Build history of the part. All positions in model axes, mm. Face numbers are marked on the shaded views. A direction names the side the tool comes from. Round coordinates to 2 decimals unless told otherwise and drop trailing zeros. Write each loop counter-clockwise with the first axis right and the second up, starting at its lowest first coordinate (ties: lowest second). Pieces come first, ordered by that corner, then holes. Notation, with made-up numbers: (83.5, 0) - (136.5, 0) arc R15 cw to (136.5, 24) - close; hole circle Ø3 at (53.25, -12.75). An arc over 180 degrees is marked (long way). Answer as a JSON object with one key per item and string values. Group by question number.
Item 1: Flat gauge pins, fed straight in: pin 1 (0.5 mm diameter, centred on y = 5.5, z = 0, fed in from +X); pin 2 (1.2 mm diameter, centred on x = -4, z = 1, fed in from -Y); pin 3 (1.5 mm diameter, centred on x = -3.5, y = 3.5, fed in from -Z). Where does each tip first touch, or does it go through?
Item 2: Which spindle directions (+Z, -Z, +X, -X, +Y, -Y) get a long thin tool onto all of the face, cutting with end or side? Do the marked faces 1, 2, 3 and 4. Say none if no direction does.
Item 3: Slice it at A-A, the plane x = -4.6. List the corners of the cut face in (y, z).
Item 4: Slice it at B-B, the plane y = -3.75. List the corners of the cut face in (x, z).
Item 5: Slice it at C-C, the plane z = -1.65. List the corners of the cut face in (x, y), then the cut area to 3 significant figures.
Item 6: Two-plate mould, pull along Y, no slides. Class the marked faces 5, 6 and 7: +Y half, -Y half, draft (parallel to the pull), parting line (faces both ways), or undercut.
Item 7: Probe line 1 (X direction, y = -3.7, z = 0); line 2 (Y direction, x = 0, z = 1.25); line 3 (Y direction, x = -3.25, z = 0.8). List the from-to ranges inside material, lowest first. Write a range as from..to.
Item 8: Slice it at D-D, the plane x = 0. List the corners of the cut face in (y, z).
from build123d import *

# Parameters (mm, degrees)
EXTRUDE_1_DEPTH      = 4
EXTRUDE_1_DEPTH_BACK = 4
SKETCH_1_R           = 0.75
SKETCH_2_R           = 2
EXTRUDE_2_DEPTH      = 1
EXTRUDE_START        = 1
SKETCH_3_R           = 2
EXTRUDE_3_DEPTH      = 1
SKETCH_4_W           = 2
SKETCH_4_H           = 2
EXTRUDE_4_DEPTH      = 0.75
SKETCH_5_W           = 2
SKETCH_5_H           = 2
EXTRUDE_5_DEPTH      = 0.75
SKETCH_6_W           = 1.5
SKETCH_6_H           = 3
EXTRUDE_6_DEPTH      = 1
SKETCH_7_W           = 1.5
SKETCH_7_H           = 3
EXTRUDE_8_DEPTH      = 1
SKETCH_8_W           = 3
SKETCH_8_H           = 2
EXTRUDE_9_DEPTH      = 0.5
EXTRUDE_10_DEPTH     = 1
EXTRUDE_START_2      = 7
EXTRUDE_11_DEPTH     = 1
CUT_EXTRUDE_1_DEPTH  = 12.942466244
FILLET_1_R           = 0.1


with BuildPart() as part:
    # 草图1 → 凸台-拉伸1 (new, two sides: drawn at the far end of the back side and taken through both)
    with BuildSketch(Plane(origin=(0, 0, 0), x_dir=(1, 0, 0), z_dir=(0, 1, 0)).offset(-EXTRUDE_1_DEPTH_BACK)):
        with Locations(Location((0, 0, 0), (0, 0, 270))):
            Circle(SKETCH_1_R)
    extrude(amount=EXTRUDE_1_DEPTH + EXTRUDE_1_DEPTH_BACK)

    # 草图2 → 凸台-拉伸2 (add)
    with BuildSketch(Plane(origin=(0, 4, 0), x_dir=(-1, 0, 0), z_dir=(0, 1, 0))):
        with Locations(Location((0, 0, 0), (0, 0, 90))):
            Circle(SKETCH_2_R)
    extrude(amount=EXTRUDE_2_DEPTH)

    # 草图3 → 凸台-拉伸3 (add)
    with BuildSketch(Plane.XZ.offset(4).offset(EXTRUDE_START)):
        with Locations(Location((0, 0, 0), (0, 0, 90))):
            Circle(SKETCH_3_R)
    extrude(amount=-EXTRUDE_3_DEPTH)

    # 草图4 → 凸台-拉伸4 (add)
    with BuildSketch(Plane(origin=(0, 5, 0), x_dir=(-1, 0, 0), z_dir=(0, 1, 0))):
        Rectangle(SKETCH_4_W, SKETCH_4_H)
    extrude(amount=EXTRUDE_4_DEPTH)

    # 草图5 → 凸台-拉伸5 (add)
    with BuildSketch(Plane.XZ.offset(5)):
        Rectangle(SKETCH_5_W, SKETCH_5_H)
    extrude(amount=EXTRUDE_5_DEPTH)

    # 草图6 → 凸台-拉伸6 (add)
    with BuildSketch(Plane(origin=(0, 5, 0), x_dir=(-1, 0, 0), z_dir=(0, 1, 0))):
        with Locations((1.75, 0)):
            Rectangle(SKETCH_6_W, SKETCH_6_H)
    extrude(amount=-EXTRUDE_6_DEPTH)

    # 草图7 → 凸台-拉伸8 (add)
    with BuildSketch(Plane.XZ.offset(5)):
        with Locations((-1.75, 0)):
            Rectangle(SKETCH_7_W, SKETCH_7_H)
    extrude(amount=-EXTRUDE_8_DEPTH)

    # 草图8 → 凸台-拉伸9 (add)
    with BuildSketch(Plane.ZY.offset(2.5)):
        with Locations((0, 4)):
            Rectangle(SKETCH_8_W, SKETCH_8_H)
        with Locations((0, -4)):
            Rectangle(SKETCH_8_W, SKETCH_8_H)
    extrude(amount=-EXTRUDE_9_DEPTH)

    # 草图9 → 凸台-拉伸10 (add)
    with BuildSketch(Plane.XZ.offset(-3)):
        with BuildLine():
            Line((-2.5, -1.5), (-3.277124344, -1.5))
            ThreePointArc((-3.277124344, -1.5), (-6.6, 0), (-3.277124344, 1.5))
            Line((-3.277124344, 1.5), (-2.5, 1.5))
            Line((-2.5, 1.5), (-2.5, -1.5))
        make_face()
    extrude(amount=-EXTRUDE_10_DEPTH)

    # 草图9<2> → 凸台-拉伸11 (add)
    with BuildSketch(Plane.XZ.offset(-3).offset(EXTRUDE_START_2)):
        with BuildLine():
            Line((-2.5, -1.5), (-3.277124344, -1.5))
            ThreePointArc((-3.277124344, -1.5), (-6.6, 0), (-3.277124344, 1.5))
            Line((-3.277124344, 1.5), (-2.5, 1.5))
            Line((-2.5, 1.5), (-2.5, -1.5))
        make_face()
    extrude(amount=-EXTRUDE_11_DEPTH)

    # 草图10 → 切除-拉伸1 (cut, through all)
    with BuildSketch(Plane(origin=(0, 4, 0), x_dir=(-1, 0, 0), z_dir=(0, 1, 0))):
        with BuildLine():
            Line((5.35, 0), (5.35, -1.854049622))
            ThreePointArc((5.35, -1.854049622), (4.548070298, -1.999325713), (3.754763477, -1.812615574))
            Line((3.754763477, -1.812615574), (4.283036304, -0.67973084))
            ThreePointArc((4.283036304, -0.67973084), (4.197025294, 0.632543584), (5.35, 0))
        make_face()
    extrude(amount=-CUT_EXTRUDE_1_DEPTH, mode=Mode.SUBTRACT)

    # 圆角1
    fillet_1_edges = [part.edges().sort_by_distance(p)[0] for p in [
        (1, 5.375, 1),
        (1, 5.375, -1),
        (-1, 5.375, -1),
        (-1, 5.375, 1),
        (1, 5.75, 0),
        (0, 5.75, -1),
        (-1, 5.75, 0),
        (0, 5.75, 1),
        (-1, -5.375, 1),
        (-1, -5.375, -1),
        (1, -5.375, -1),
        (1, -5.375, 1),
        (-1, -5.75, 0),
        (0, -5.75, -1),
        (1, -5.75, 0),
        (0, -5.75, 1),
    ]]
    fillet(fillet_1_edges, radius=FILLET_1_R)


solid = part.part
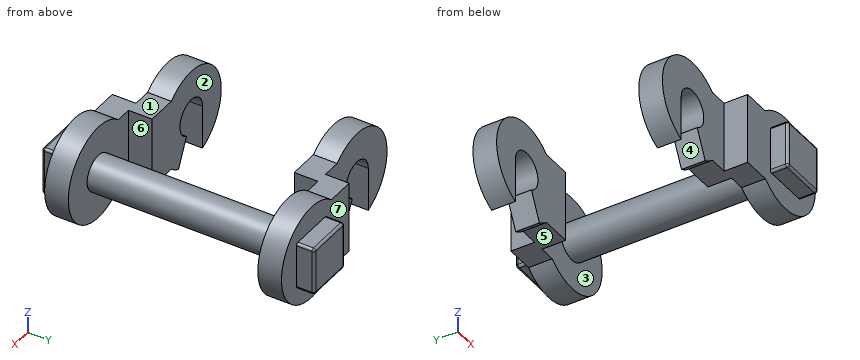
Geometry says:
{
 "1": {"pin 1": "stops at x = 1", "pin 2": "stops at y = -4", "pin 3": "stops at z = -1.81"},
 "2": {"face 1": "+Z, +Y, -Y", "face 2": "+Z, -Z, -X", "face 3": "none", "face 4": "-Z, +Y, -Y"},
 "3": {"outline": "(-4, 0.75) - (-3, 0.75) - (-3, 2) - (-4, 2) - close; (3, 0.75) - (4, 0.75) - (4, 2) - (3, 2) - close"},
 "4": {"outline": "(-5.35, -1.85) - (-5.35, 0) arc R0.75 cw (long way) to (-4.28, -0.68) - (-3.75, -1.81) arc R2 ccw to (-3.28, -1.5) - (-2, -1.5) - (-2, 1.5) - (-3.28, 1.5) arc R2 ccw (long way) to start; circle Ø1.5 at (0, 0)"},
 "5": {"outline": "(-5.73, -4) - (-5.35, -4) - (-5.35, -3) - (-5.73, -3) - close; (-5.73, 3) - (-5.35, 3) - (-5.35, 4) - (-5.73, 4) - close; (-3.83, -4) - (-3.47, -4) - (-3.47, -3) - (-3.83, -3) - close; (-3.83, 3) - (-3.47, 3) - (-3.47, 4) - (-3.83, 4) - close; (-1.13, -5) - (1.13, -5) - (1.13, -4) - (-1.13, -4) - close; (-1.13, 4) - (1.13, 4) - (1.13, 5) - (-1.13, 5) - close", "area": "6.00 mm^2"},
 "6": {"face 5": "draft", "face 6": "undercut", "face 7": "+Y half"},
 "7": {"line 1": "x = -6.6..-5.35, -3.85..-2, -0.75..0.75", "line 2": "y = -5..-4, 4..5", "line 3": "y = -4..-3, 3..4"},
 "8": {"outline": "(-5.75, -0.9) arc R0.1 ccw to (-5.65, -1) - (-5, -1) - (-5, -2) - (-4, -2) - (-4, -0.75) - (4, -0.75) - (4, -2) - (5, -2) - (5, -1) - (5.65, -1) arc R0.1 ccw to (5.75, -0.9) - (5.75, 0.9) arc R0.1 ccw to (5.65, 1) - (5, 1) - (5, 2) - (4, 2) - (4, 0.75) - (-4, 0.75) - (-4, 2) - (-5, 2) - (-5, 1) - (-5.65, 1) arc R0.1 ccw to (-5.75, 0.9) - close"}
}
